from build123d import *

# Parameters (mm, degrees)
F1_DEPTH = 13.5
F2_R     = 6.74999
F3_R     = 3
F4_W     = 12.2435482951
F4_H     = 30
F5_DEPTH = 14
F6_R     = 4


# Not quite as in the source:
# - a fillet or chamfer is up to 0.001 mm smaller than in the source, because OpenCascade refuses the exact size


with BuildPart() as f1:
    # F0 (on Front) → F1 (new body)
    with BuildSketch(Plane.XZ):
        Polygon((0, 26), (0, 0), (17, 0), (25, -8.16), (34, -8.16), (34, 8.34), (24, 8.34), (10, 26), align=None)
    extrude(amount=F1_DEPTH)

    # F2 (radius 6.75 in the source; OpenCascade refuses exactly that, so slightly less here)
    f2_edges = [f1.edges().sort_by_distance(p)[0] for p in [
        (5, 0, 26),
        (5, -13.5, 26),
        (8.5, 0, 0),
        (8.5, -13.5, 0),
    ]]
    fillet(f2_edges, radius=F2_R)

    # F3
    f3_edges = [f1.edges().sort_by_distance(p)[0] for p in [
        (29, -13.5, 8.34),
        (29, 0, 8.34),
        (29.5, 0, -8.16),
        (29.5, -13.5, -8.16),
    ]]
    fillet(f3_edges, radius=F3_R)

    # F4 (on face) → F5 (join)
    with BuildSketch(Plane(origin=(0, 0, 0), x_dir=(-1, 0, 0), z_dir=(0, 1, 0))):
        with Locations((-28.8782258524, 4.84)):
            Rectangle(F4_W, F4_H)
    extrude(amount=F5_DEPTH)

    # F6
    f6_edges = [f1.edges().sort_by_distance(p)[0] for p in [
        (28.878226, 14, 19.84),
        (28.878226, 0, 19.84),
        (28.878226, 14, -10.16),
        (28.878226, 0, -10.16),
    ]]
    fillet(f6_edges, radius=F6_R)


solid = f1.part
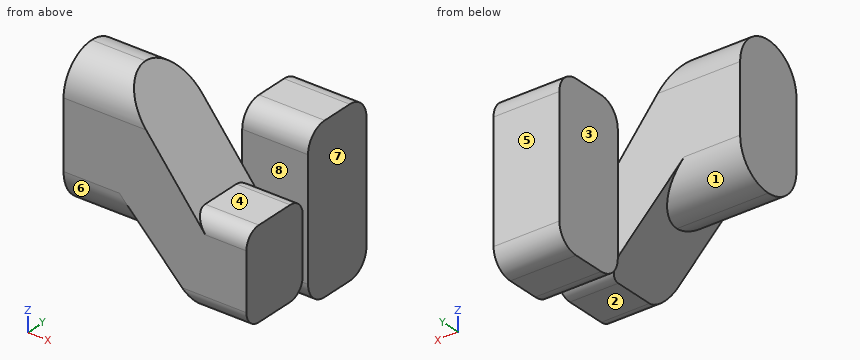
Geometry: final body of the model. Coordinates: model frame, mm. Face numbers are marked on the shaded views. A direction names the side the tool comes from. Give positions to 0.01 mm unless a question says otherwise; leave off trailing zeros. Write each loop counter-clockwise with the first axis right and the second up, starting at its lowest first coordinate (ties: lowest second). Pieces come first, ordered by that corner, then holes. Notation, with made-up numbers: (-8.75, -6.5) - (21.25, -6.5) arc R11 cw to (21.25, 14.5) - close; hole circle Ø9 at (59.25, -11.5). An arc over 180 degrees is marked (long way). Return JSON: item names as keys, results as strings. Group by question number.
1) Set-up query: the marked faces 1, 2, 3 and 4. Return all of +Z, -Z, +X, -X, +Y, -Y with unobstructed straight access to the full face (end or side cutting, diameter ignored); none if empty.
2) Mould query, pull axis Y, two halves, no side actions, for the marked faces 5, 6, 7 and 8. Classes: released by +Y, released by -Y, zero draft, split by the parting line, or undercut.
3) Section C-C on y = -5.5. Return the cut outline in (x, z).
4) Section A-A on x = 27. Return the cut outline in (y, z), plus the area to 3 significant figures.
5) Line query: line 1 (Y direction, x = 15, z = 13); line 2 (Z direction, x = 30.5, y = -2.75); line 3 (X direction, y = -0.5, z = 0). Output: solid intervals per line, ascending.
6) First-contact query: P1, Ø7, axis at y = -10, z = 2.5, coming from the +X side; P2, Ø4, axis at x = 29.5, y = -8.5, coming from the +Z side; P3, Ø4, axis at x = 22.5, z = 18, coming from the +Y side. Flat tips, straight axial feed; report the tip coordinate or a pass-through.
7) Section B-B on z = 9. Return the cut outline in (x, y), plus the area to 3 significant figures.
8) Section D-D on z = 1. Return the cut outline in (x, y).
Filled in:
{
 "1": {"face 1": "-Z, -X, +Y", "face 2": "-Z, +X, -X, -Y", "face 3": "+Z, -Z, -X, +Y", "face 4": "+Z, +X, -Y"},
 "2": {"face 5": "released by +Y", "face 6": "released by -Y", "face 7": "zero draft", "face 8": "undercut"},
 "3": {"outline": "(0, 0.12) - (16.89, 0.12) - (25, -8.16) - (34, -8.16) - (34, 8.34) - (24, 8.34) - (10.09, 25.88) - (0, 25.88) - close"},
 "4": {"outline": "(-13.5, -5.16) arc R3 ccw to (-10.5, -8.16) - (-3, -8.16) arc R3 ccw to (0, -5.16) - (0, -6.16) arc R4 ccw to (4, -10.16) - (10, -10.16) arc R4 ccw to (14, -6.16) - (14, 15.84) arc R4 ccw to (10, 19.84) - (4, 19.84) arc R4 ccw to (0, 15.84) - (0, 5.34) arc R3 ccw to (-3, 8.34) - (-10.5, 8.34) arc R3 ccw to (-13.5, 5.34) - close", "area": "621 mm^2"},
 "5": {"line 1": "y = -13.5 to 0", "line 2": "z = -8.15 to 8.33", "line 3": "x = 17 to 34"},
 "6": {"P1": "stops at x = 34", "P2": "stops at z = 8.34", "P3": "stops at y = 14"},
 "7": {"outline": "(0, -13.5) - (23.48, -13.5) - (23.48, 0) - (35, 0) - (35, 14) - (22.76, 14) - (22.76, 0) - (0, 0) - close", "area": "488 mm^2"},
 "8": {"outline": "(0, -10.29) - (16.02, -10.29) - (16.02, -13.5) - (34, -13.5) - (34, 0) - (35, 0) - (35, 14) - (22.76, 14) - (22.76, 0) - (16.02, 0) - (16.02, -3.21) - (0, -3.21) - close"}
}
